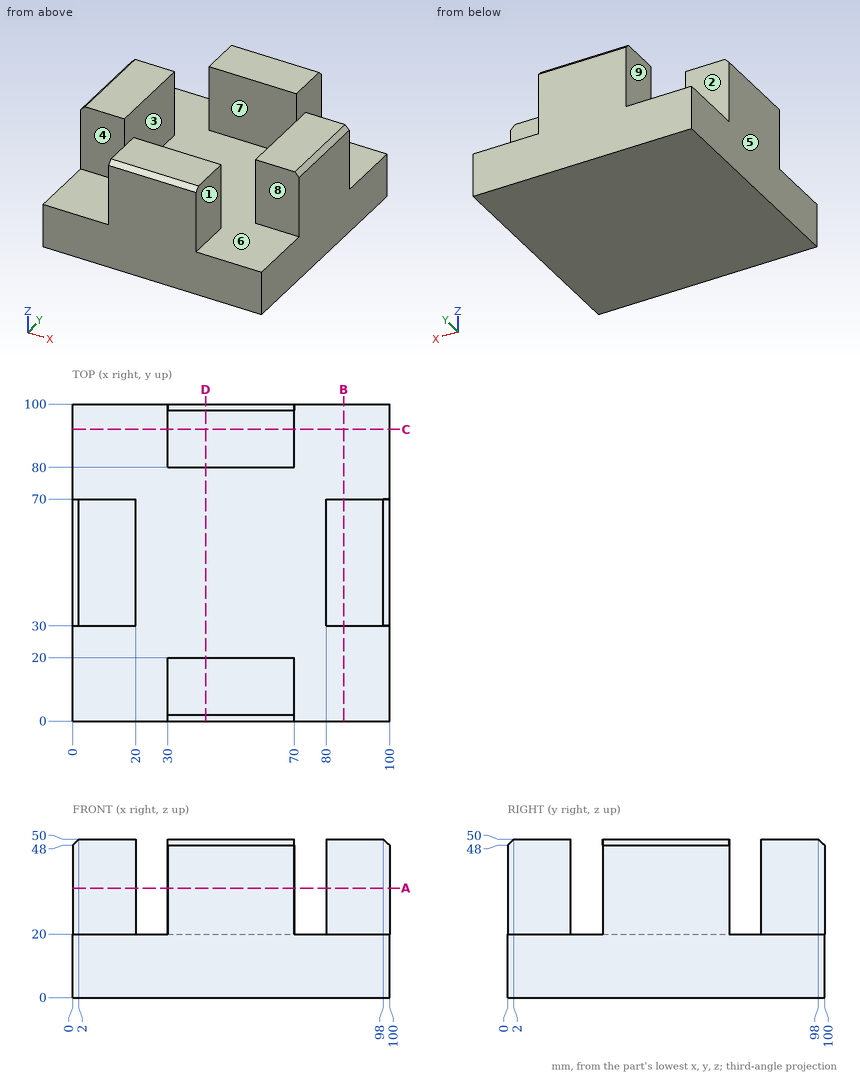
Here's the drawing with two shaded views (mm, measured from the low corner). I have some questions. A direction names the side the tool comes from. Round coordinates to 2 decimals unless told otherwise and drop trailing zeros. Order: outer loops, then holes, each group sorted by start corner. A loop starts at its lowest first (then second) coordinate and runs counter-clockwise, first axis right, second up. Notation, with made-up numbers: M -30,53 L 6,53 A32 cw 6,91 Z; hole C 57.5,22.5 d10. An arc over 180 degrees is marked long. Use CSV: the item, a comma, the result in double quotes.
1) If we mould it in two halves opening along Y, with no side actions, what happens to the marked faces 6, 7, 8 and 9? For each: pulls with the +Y half, pulls with the -Y half, needs draft (parallel to the pull), parting line crosses it, or undercut.
Taken from the geometry:
face 6,"undercut"
face 7,"undercut"
face 8,"pulls with the -Y half"
face 9,"needs draft"
2) I'm going to push flat-ended pins straight in: P1, Ø5, axis at x = 11.5, y = 55, coming from the -Z side; P2, Ø5, axis at x = 23.5, y = 85.5, coming from the +Z side; P3, Ø10, axis at x = 94.5, z = 41, coming from the +Y side; P4, Ø16, axis at y = 5.5, z = 29.5, coming from the -X side. Where does each tip first touch, or does it pass through?
Taken from the geometry:
P1,"z = 0"
P2,"z = 20"
P3,"y = 70"
P4,"x = 30"
3) I want a section at D-D (x = 42). List the corners of the cut face in (y, z) for me.
Taken from the geometry:
outline,"M 0,0 L 100,0 L 100,48 L 98,50 L 80,50 L 80,20 L 20,20 L 20,50 L 2,50 L 0,48 Z"
4) I want a section at B-B (x = 85.5). List the corners of the cut face in (y, z) for me.
Taken from the geometry:
outline,"M 0,0 L 100,0 L 100,20 L 70,20 L 70,50 L 30,50 L 30,20 L 0,20 Z"
5) On a 3-axis mill with a long thin cutter (end or side, diameter ignored), from which of +Z, -Z, +X, -X, +Y, -Y can I reach the whole of each face in a straight line? I mean the marked faces 1, 2, 3, 4 and 5. Say none if no direction works.
Taken from the geometry:
face 1,"+Z, +X, +Y, -Y"
face 2,"+Z, +X, -X, +Y"
face 3,"+Z, +Y, -Y"
face 4,"+Z, +X, -X, -Y"
face 5,"+Z, -Z, -X, +Y, -Y"
6) I need wall thicknesses on line 1 along Y through (x, z) = (42.5, 37.5); line 2 along Z through (x, y) = (23.5, 67.5). Which ranges of each line are inside material? Lowest first, please. Write a range as [from, to].
Taken from the geometry:
line 1,"[0, 20], [80, 100]"
line 2,"[0, 20]"
7) I want a section at A-A (z = 34.5). List the corners of the cut face in (x, y) for me.
Taken from the geometry:
outline,"M 0,30 L 20,30 L 20,70 L 0,70 Z; M 30,0 L 70,0 L 70,20 L 30,20 Z; M 30,80 L 70,80 L 70,100 L 30,100 Z; M 80,30 L 100,30 L 100,70 L 80,70 Z"
